from build123d import *

# Parameters (mm, degrees)
SKETCH1_W           = 52.5
SKETCH1_H           = 18.8
BOSS_EXTRUDE1_DEPTH = 1
BOSS_EXTRUDE2_DEPTH = 4
BOSS_EXTRUDE3_DEPTH = 14
FILLET1_R           = 2
FILLET2_R           = 2
FILLET3_R           = 1


with BuildPart() as part:
    # Sketch1 → Boss-Extrude1 (new body)
    with BuildSketch(Plane.XY):
        Rectangle(SKETCH1_W, SKETCH1_H)
    extrude(amount=BOSS_EXTRUDE1_DEPTH)

    # Sketch2 → Boss-Extrude2 (add, symmetric)
    with BuildSketch(Plane(origin=(0, 0, 0), x_dir=(1, 0, 0), z_dir=(0, 1, 0))):
        with BuildLine():
            Line((-26.25, 0), (-26.25, -1))
            ThreePointArc((-26.25, -1), (-26.547428998, -8.015097806), (-25.75, -14.99106858))
            ThreePointArc((-25.75, -14.99106858), (-26.232288437, -17.75177498), (-27.713282794, -15.372540297))
            ThreePointArc((-27.713282794, -15.372540297), (-28.546153081, -8.086526378), (-28.235505016, -0.759646447))
            Line((-28.235505016, -0.759646447), (-28.235505016, 0))
            Line((-28.235505016, 0), (-26.25, 0))
        make_face()
    boss_extrude2 = extrude(amount=BOSS_EXTRUDE2_DEPTH, both=True)

    # Mirror1: Boss-Extrude2 across plane
    add(boss_extrude2.mirror(Plane(origin=(0, 0, 0), x_dir=(0, 0, 1), z_dir=(1, 0, 0))))

    # Sketch3 → Boss-Extrude3 (add, symmetric)
    with BuildSketch(Plane(origin=(0, 0, 0), x_dir=(0, 0, -1), z_dir=(1, 0, 0))):
        with BuildLine():
            Line((0, 9.4), (-1, 9.4))
            ThreePointArc((-1, 9.4), (-8.019576143, 9.698132003), (-15, 8.9))
            ThreePointArc((-15, 8.9), (-17.760743831, 9.382074127), (-15.381624121, 10.863253175))
            ThreePointArc((-15.381624121, 10.863253175), (-8.090959204, 11.696857712), (-0.759401899, 11.385475397))
            Line((-0.759401899, 11.385475397), (0, 11.385475397))
            Line((0, 11.385475397), (0, 9.4))
        make_face()
    boss_extrude3 = extrude(amount=BOSS_EXTRUDE3_DEPTH, both=True)

    # Mirror2: Boss-Extrude3 across plane
    add(boss_extrude3.mirror(Plane.ZX))

    # Fillet1
    fillet1_edges = [part.edges().sort_by_distance(p)[0] for p in [
        (0, 9.4, 1),
        (-26.25, 0, 1),
        (0, -9.4, 1),
        (26.25, 0, 1),
        (26.25, -9.4, 0.5),
        (26.25, 9.4, 0.5),
        (-26.25, -9.4, 0.5),
        (-26.25, 9.4, 0.5),
    ]]
    fillet(fillet1_edges, radius=FILLET1_R)

    # Fillet2
    # the kernel refuses this fillet: 2 mm, written as the material it adds along each edge
    with BuildSketch(Plane(origin=(-14, -9.4, 0), x_dir=(0, -1, 0), z_dir=(0, 0, 1))) as fillet2_piece_1_section:
        with BuildLine():
            CenterArc((FILLET2_R, -FILLET2_R), FILLET2_R, 90, 90)
            Line((0, -FILLET2_R), (0, 0))
            Line((0, 0), (FILLET2_R, 0))
        make_face()
    fillet2_piece_1 = extrude(amount=1, mode=Mode.PRIVATE)
    fillet2_piece_1 = split(fillet2_piece_1, bisect_by=Plane(origin=(-14.000636708, -11.385475397, 0.169006007), z_dir=(0, 1, 0)), keep=Keep.TOP, mode=Mode.PRIVATE)
    add(fillet2_piece_1)
    with BuildSketch(Plane(origin=(-14, -9.4, -5), x_dir=(0, -1, 0), z_dir=(0, 0, 1))) as fillet2_piece_2_section:
        with BuildLine():
            CenterArc((FILLET2_R, -FILLET2_R), FILLET2_R, 90, 90)
            Line((0, -FILLET2_R), (0, 0))
            Line((0, 0), (FILLET2_R, 0))
        make_face()
    fillet2_piece_2 = extrude(amount=6, mode=Mode.PRIVATE)
    fillet2_piece_2 = split(fillet2_piece_2, bisect_by=Plane(origin=(-14.000016578, -11.385475397, 0.893450241), z_dir=(0, -1, 0)), keep=Keep.TOP, mode=Mode.PRIVATE)
    fillet2_piece_2 = fillet2_piece_2 & Plane(origin=(-14.000016578, 35.273196442, 6.41345727), x_dir=(0, -0.9816265876102759, 0.19081206066862103), z_dir=(1, 0, 0)) * Cylinder(47, 21, mode=Mode.PRIVATE)
    add(fillet2_piece_2)
    with BuildSketch(Plane(origin=(14, -9.4, 0), x_dir=(1, 0, 0), z_dir=(0, 0, 1))) as fillet2_piece_3_section:
        with BuildLine():
            CenterArc((FILLET2_R, -FILLET2_R), FILLET2_R, 90, 90)
            Line((0, -FILLET2_R), (0, 0))
            Line((0, 0), (FILLET2_R, 0))
        make_face()
    fillet2_piece_3 = extrude(amount=1, mode=Mode.PRIVATE)
    fillet2_piece_3 = split(fillet2_piece_3, bisect_by=Plane(origin=(14.446749005, -11.385475397, 0.500009641), z_dir=(0, 1, 0)), keep=Keep.TOP, mode=Mode.PRIVATE)
    add(fillet2_piece_3)
    with BuildSketch(Plane(origin=(14, -9.4, -5), x_dir=(1, 0, 0), z_dir=(0, 0, 1))) as fillet2_piece_4_section:
        with BuildLine():
            CenterArc((FILLET2_R, -FILLET2_R), FILLET2_R, 90, 90)
            Line((0, -FILLET2_R), (0, 0))
            Line((0, 0), (FILLET2_R, 0))
        make_face()
    fillet2_piece_4 = extrude(amount=6, mode=Mode.PRIVATE)
    fillet2_piece_4 = split(fillet2_piece_4, bisect_by=Plane(origin=(14.000016578, -11.385475397, 0.893450335), z_dir=(0, -1, 0)), keep=Keep.TOP, mode=Mode.PRIVATE)
    fillet2_piece_4 = fillet2_piece_4 & Plane(origin=(14.000016578, 35.273196442, 6.41345727), x_dir=(0, -0.9816265876102759, 0.19081206066862103), z_dir=(1, 0, 0)) * Cylinder(47, 20, mode=Mode.PRIVATE)
    add(fillet2_piece_4)
    with BuildSketch(Plane(origin=(14, 9.4, 0), x_dir=(1, 0, 0), z_dir=(0, 0, 1))) as fillet2_piece_5_section:
        with BuildLine():
            CenterArc((FILLET2_R, FILLET2_R), FILLET2_R, 180, 90)
            Line((0, FILLET2_R), (0, 0))
            Line((0, 0), (FILLET2_R, 0))
        make_face()
    fillet2_piece_5 = extrude(amount=1, mode=Mode.PRIVATE)
    fillet2_piece_5 = split(fillet2_piece_5, bisect_by=Plane(origin=(14.446749005, 11.385475397, 0.500009641), z_dir=(0, -1, 0)), keep=Keep.TOP, mode=Mode.PRIVATE)
    add(fillet2_piece_5)
    with BuildSketch(Plane(origin=(14, 9.4, -5), x_dir=(1, 0, 0), z_dir=(0, 0, 1))) as fillet2_piece_6_section:
        with BuildLine():
            CenterArc((FILLET2_R, FILLET2_R), FILLET2_R, 180, 90)
            Line((0, FILLET2_R), (0, 0))
            Line((0, 0), (FILLET2_R, 0))
        make_face()
    fillet2_piece_6 = extrude(amount=6, mode=Mode.PRIVATE)
    fillet2_piece_6 = split(fillet2_piece_6, bisect_by=Plane(origin=(14.000016578, 11.385475397, 0.893450335), z_dir=(0, 1, 0)), keep=Keep.TOP, mode=Mode.PRIVATE)
    fillet2_piece_6 = fillet2_piece_6 & Plane(origin=(14.000016578, -35.273196442, 6.41345727), x_dir=(0, 0.9816265876102759, 0.19081206066862103), z_dir=(1, 0, 0)) * Cylinder(47, 21, mode=Mode.PRIVATE)
    add(fillet2_piece_6)
    with BuildSketch(Plane(origin=(-14, 9.4, 0), x_dir=(0, 1, 0), z_dir=(0, 0, 1))) as fillet2_piece_7_section:
        with BuildLine():
            CenterArc((FILLET2_R, FILLET2_R), FILLET2_R, 180, 90)
            Line((0, FILLET2_R), (0, 0))
            Line((0, 0), (FILLET2_R, 0))
        make_face()
    fillet2_piece_7 = extrude(amount=1, mode=Mode.PRIVATE)
    fillet2_piece_7 = split(fillet2_piece_7, bisect_by=Plane(origin=(-14.000636708, 11.385475397, 0.169006007), z_dir=(0, -1, 0)), keep=Keep.TOP, mode=Mode.PRIVATE)
    add(fillet2_piece_7)
    with BuildSketch(Plane(origin=(-14, 9.4, -5), x_dir=(0, 1, 0), z_dir=(0, 0, 1))) as fillet2_piece_8_section:
        with BuildLine():
            CenterArc((FILLET2_R, FILLET2_R), FILLET2_R, 180, 90)
            Line((0, FILLET2_R), (0, 0))
            Line((0, 0), (FILLET2_R, 0))
        make_face()
    fillet2_piece_8 = extrude(amount=6, mode=Mode.PRIVATE)
    fillet2_piece_8 = split(fillet2_piece_8, bisect_by=Plane(origin=(-14.000016578, 11.385475397, 0.893450241), z_dir=(0, 1, 0)), keep=Keep.TOP, mode=Mode.PRIVATE)
    fillet2_piece_8 = fillet2_piece_8 & Plane(origin=(-14.000016578, -35.273196442, 6.41345727), x_dir=(0, 0.9816265876102759, 0.19081206066862103), z_dir=(1, 0, 0)) * Cylinder(47, 20, mode=Mode.PRIVATE)
    add(fillet2_piece_8)

    # Fillet3
    fillet3_edges = [part.edges().sort_by_distance(p)[0] for p in [
        (-27.713282794, 0, 15.372540297),
        (27.713282794, 0, 15.372540297),
        (0, 10.863253175, 15.381624121),
        (0, -10.863253175, 15.381624121),
    ]]
    fillet(fillet3_edges, radius=FILLET3_R)


solid = part.part
Geometry check sheet. Reference: the model listing, model coordinates, mm. A direction names the side the tool comes from. Round coordinates to 2 decimals unless told otherwise and drop trailing zeros. Order: outer loops, then holes, each group sorted by start corner. A loop starts at its lowest first (then second) coordinate and runs counter-clockwise, first axis right, second up. Notation, with made-up numbers: (-18.75, -30.75) - (-7.75, -30.75) arc R18 cw to (-7.75, -9.75) - close; hole circle Ø8 at (48, 1). An arc over 180 degrees is marked (long way). One line per question, with ' | ' between items. Start each with the question number.
(1) Thickness scan on L1, parallel to Y at x = 4.5, z = 7.25; L2, parallel to Z at x = -1.5, y = -7.75; L3, parallel to X at y = 3, z = 9.25. Record the ranges inside material, lowest first. Write a range as [from, to].
(2) Sectioned sample at C-C on z = 3.5. Record the cut outline in (x, y).
(3) Sectioned sample at D-D on x = -15. Record the cut outline in (y, z).
(4) Release check for a two-part mould opening along Z. For faces 6 (the flat face through (0, 0, 1)), 7 (the cylindrical face through (0.2, 9.19, 17.71)), 8 (the flat face through (-14, 10, 9)) record: released by +Z, released by -Z, zero draft, split by the parting line, or undercut.
(5) Access from +Z, -Z, +X, -X, +Y, -Y to the whole of each face (thin tool, end or side, straight path). Record for faces 1 (the flat face through (14, 10, 9)), 2 (the cylindrical face through (25.782, -0.056, 1.517)), 3 (the flat face through (-20.2, -9.4, 0.5)), 4 (the cylindrical face through (-0.196, 8.933, 1.517)), 5 (the flat face through (26.25, -5.7, 0.5)).
(6) Depth check by flat-ended pin: pin 1 Ø10 at (x, z) = (14.5, 13) entering from -Y; pin 2 Ø4 at (y, z) = (4.5, 5) entering from -X; pin 3 Ø8 at (x, z) = (8.5, 11.5) entering from +Y. Enter the tip coordinate at first touch or a pass-through.
(7) Sectioned sample at B-B on y = -5.25. Record the cut outline in (x, z).
(8) Sectioned sample at A-A on z = 7.25. Record the cut outline in (x, y), and give its area (3 significant figures).
Conclusion:
1) L1: y = [-11.72, -9.72], [9.72, 11.72] | L2: z = [0, 1.01] | L3: x = [-28.49, -26.49], [26.49, 28.49]
2) outline: (-28.49, -4) - (-26.48, -4) - (-26.48, 4) - (-28.49, 4) - close; (-14, -11.64) - (14, -11.64) - (14, -9.63) - (-14, -9.63) - close; (-14, 9.63) - (14, 9.63) - (14, 11.64) - (-14, 11.64) - close; (26.48, -4) - (28.49, -4) - (28.49, 4) - (26.48, 4) - close
3) outline: (-9.67, 0) - (9.67, 0) - (9.67, 1) - (-9.67, 1) - close
4) face 6: released by +Z | face 7: undercut | face 8: zero draft
5) face 1: +Z, +X, +Y, -Y | face 2: +Y, -Y | face 3: +Z, -Z, -X, -Y | face 4: +X, -X | face 5: +Z, -Z, +X, -Y
6) pin 1: stops at y = -11.7 | pin 2: stops at x = -28.58 | pin 3: stops at y = 11.71
7) outline: (-26.25, 0) - (26.25, 0) - (26.25, 1) - (-26.25, 1) - close
8) outline: (-28.57, -4) - (-26.57, -4) - (-26.57, 4) - (-28.57, 4) - close; (-14, -11.72) - (14, -11.72) - (14, -9.72) - (-14, -9.72) - close; (-14, 9.72) - (14, 9.72) - (14, 11.72) - (-14, 11.72) - close; (26.57, -4) - (28.57, -4) - (28.57, 4) - (26.57, 4) - close | area: 144 mm2
